Autodesk Inventor part; units mm, degrees
ref_plane "YZ Plane" through (0, 0, 0) normal (1, 0, 0) x (0, 1, 0)
ref_plane "XZ Plane" through (0, 0, 0) normal (0, 1, 0) x (-1, 0, 0)
ref_plane "XY Plane" through (0, 0, 0) normal (0, 0, 1) x (1, 0, 0)
sketch "Sketch1" plane through (0, 0, 0) normal (1, 0, 0) x (0, 1, 0)
  line L0 (-25, 24) -> (-25, -24)
  line L1 (-25, -24) -> (25, -24)
  line L2 (25, -24) -> (25, -22)
  line L3 (25, -22) -> (-23, -22)
  line L4 (-23, -22) -> (-23, 24)
  line L5 (-23, 24) -> (-25, 24)
extrude "Extrusion1" add sketch "Sketch1" along normal mid plane 131
sketch "Sketch2" plane through (65.5, 25, -24) normal (0, 0, -1) x (-1, 0, 0)
  circle A0 centre (41.4, -25) radius 3.5
  circle A1 centre (89.6, -25) radius 3.5
  line L0 (131, 0) -> (0, 0)
  line L1 (37.9, -25) -> (44.9, -25)
  line L2 (44.9, -25) -> (44.9, 0)
  line L3 (44.9, 0) -> (37.9, 0)
  line L4 (37.9, 0) -> (37.9, -25)
  line L5 (86.1, -25) -> (93.1, -25)
  line L6 (93.1, -25) -> (93.1, 0)
  line L7 (93.1, 0) -> (86.1, 0)
  line L8 (86.1, 0) -> (86.1, -25)
  line L9 (65.5, 0) -> (65.5, -8)
  circle A2 centre (65.5, -8) radius 4.75
  dimension "d17" = 7
  dimension "d18" = 7
  dimension "d129" = 8
  dimension "d130" = 9.5
hole "Hole1" at (24.1, 0, -24) at (-24.1, 0, -24) direction (0, 0, 1) diameter 7 depth 2
sketch "Sketch3" plane through (65.5, 25, -24) normal (0, 0, -1) x (-1, 0, 0)
  line L0 (65.5, -25) -> (14.2, -25)
  line L1 (65.5, -25) -> (116.8, -25)
  circle A0 centre (14.2, -25) radius 9.5
  circle A1 centre (14.2, -25) radius 1.75
  circle A2 centre (116.8, -25) radius 1.75
  dimension "d26" = 51.3
  dimension "d27" = 51.3
  dimension "d28" = 19
  dimension "d29" = 3.5
  dimension "d30" = 3.5
hole "Hole2" at (51.3, 0, -24) at (-51.3, 0, -24) direction (0, 0, 1) diameter 3.5 depth 2
sketch "Sketch7" plane through (65.5, 25, -24) normal (0, 0, -1) x (-1, 0, 0)
  circle A0 centre (14.2, -25) radius 1.75
  circle A1 centre (14.2, -25) radius 3.5
  point P0 (65.5, -25)
  dimension "d89" = 7
extrude "Extrusion3" cut sketch "Sketch7" against normal blind 2
sketch "Sketch8" plane through (65.5, 25, -24) normal (0, 0, -1) x (-1, 0, 0)
  circle A0 centre (14.2, -25) radius 3.5
  line L0 (14.2, -25) -> (39.2, -25) construction
  circle A1 centre (19.1497, -20.0503) radius 18.4
  circle A2 centre (19.1497, -20.0503) radius 15.5
  line L1 (14.2, -25) -> (19.1497, -20.0503)
  line L2 (19.1497, -20.0503) -> (36.8274, -2.3726)
  line L3 (36.8274, -2.3726) -> (1.4721, -37.7279)
  line L4 (6.139, -7.0395) -> (32.1605, -33.061)
  circle A3 centre (8.1896, -9.0901) radius 1.2
  circle A4 centre (30.1099, -31.0104) radius 1.2
  circle A5 centre (23.1614, -5.0784) radius 1.2
  circle A6 centre (4.1779, -24.0619) radius 1.2
  circle A7 centre (15.1381, -35.0221) radius 1.2
  circle A8 centre (34.1216, -16.0386) radius 1.2
  point P0 (65.5, -25)
  dimension "d96" = 31
  dimension "d97" = 25
  dimension "d98" = 180
  dimension "d99" = 50
  dimension "d100" = 2.4
  dimension "d101" = 2.4
  dimension "d104" = 2.4
  dimension "d105" = 2.4
  dimension "d106" = 2.4
  dimension "d107" = 2.4
extrude "Extrusion4" cut sketch "Sketch8" against normal blind 2 contours A3 A2 L4 | L4 A2 A3 | A4 A2 L4 | L4 A2 A4 | A6 A2 | A2 A6 | A7 A2 | A2 A7 | A8 A2 | A2 A8 | A5 A2 | A2 A5 | L4 A3 A2 | A2 A3 L4 | L4 A4 A2 | A2 A4 L4
sketch "Sketch9" plane through (65.5, 25, -24) normal (0, 0, -1) x (-1, 0, 0)
  circle A0 centre (34.1216, -16.0386) radius 1.2
  circle A1 centre (8.1896, -9.0901) radius 1.2
  circle A2 centre (15.1381, -35.0221) radius 1.2
  point P0 (65.5, -25)
extrude "Extrusion6" add sketch "Sketch9" against normal blind 2
sketch "Sketch11" plane through (65.5, 25, -24) normal (0, 0, -1) x (-1, 0, 0)
  circle A0 centre (4.1779, -24.0619) radius 1.2
  circle A1 centre (30.1099, -31.0104) radius 1.2
  circle A2 centre (23.1614, -5.0784) radius 1.2
  circle A3 centre (14.2, -25) radius 3.5
  circle A4 centre (116.8, -25) radius 1.75
  line L0 (65.5, -25) -> (65.5, 0)
  line L1 (0, 0) -> (131, 0)
  circle A5 centre (126.8221, -24.0619) radius 1.2
  circle A6 centre (100.8901, -31.0104) radius 1.2
  circle A7 centre (107.8386, -5.0784) radius 1.2
  circle A8 centre (116.8, -25) radius 3.5
extrude "Extrusion7" cut sketch "Sketch11" against normal blind 2 contours A5 | A6 | A7 | A8
sketch "Sketch12" plane through (65.5, 25, -24) normal (0, 0, -1) x (-1, 0, 0)
  circle A0 centre (116.8, -25) radius 3.5
  circle A1 centre (14.2, -25) radius 3.5
  circle A2 centre (14.2, -25) radius 6.5
  circle A3 centre (116.8, -25) radius 6.5
  point P0 (65.5, -25)
  dimension "d116" = 13
  dimension "d117" = 13
extrude "Extrusion8" cut sketch "Sketch12" against normal blind 2
extrude "Extrusion9" cut sketch "Sketch2" against normal blind 2 contours L1 A0 | L0 L6 A1 L8 | A0 L1 | A0 L4 L0 L2 | L5 A1 | A1 L5
fillet "Fillet1" radius 1 4 edges at (20.6, 25, -23) (27.6, 25, -23) (-20.6, 25, -23) (-27.6, 25, -23)
fillet "Fillet2" radius 1 2 edges at (65.5, 25, -23) (-65.5, 25, -23)
extrude "Extrusion10" cut sketch "Sketch2" against normal blind 2 contours A2
sketch "Sketch14" plane through (-65.5, -25, 24) normal (0, 0, 1) x (1, 0, 0)
  line L0 (0, 2) -> (131, 2)
  line L1 (131, 2) -> (131, 0)
  line L2 (131, 0) -> (0, 0)
  line L3 (0, 0) -> (0, 2)
  point P0 (65.5, 25)
extrude "Extrusion11" cut sketch "Sketch14" against normal blind 18
fillet "Fillet3" radius 1 2 edges at (-65.5, -24, 6) (65.5, -24, 6)
sketch "Sketch15" plane through (-65.5, -25, -24) normal (0, -1, 0) x (1, 0, 0)
  circle A0 centre (97.65, 20) radius 2
  circle A1 centre (33.35, 20) radius 2
  point P0 (65.5, 24)
  point P1 (131, 0)
  point P2 (0, 0)
  dimension "d139" = 4
  dimension "d140" = 4
extrude "Extrusion12" cut sketch "Sketch15" against normal blind 2
properties part number "drzak_motory"
Work out the finished part from the listing and answer in its coordinate system (mm). A direction names the side the tool comes from. Give positions to 0.01 mm unless a question says otherwise; leave off trailing zeros. Order: outer loops, then holes, each group sorted by start corner. A loop starts at its lowest first (then second) coordinate and runs counter-clockwise, first axis right, second up. Notation, with made-up numbers: (11, -7) -> (30, -7) arc R19 ccw to (30, 1) -> close; hole circle Ø2 at (33.5, 36.25). An arc over 180 degrees is marked (long way). Answer as CSV lines item,"result". Start each with the question number.
(1) Each of these flat-tipped pins is pushed along its axis until it touches: pin 1 Ø4 at (x, y) = (-1.5, 4.5) entering from +Z; pin 2 Ø1.5 at (x, z) = (21, -11.5) entering from +Y. Where does it stop, or does it pass through?
(2) Consider line 1 along Z through (x, y) = (32, -24); line 2 along Y through (x, z) = (-6, -10); line 3 along Z through (x, y) = (-49.5, -12.5). Determine where each line is inside the solid, lowest interval first.
(3) Which of the six approach directions +Z, -Z, +X, -X, +Y, -Y give full straight-line access (tool end or side, diameter ignored) to faces 1 (the cylindrical face through (-62.43, 0.48, -23.01)), 2 (the flat face through (-1, 1, -22))?
(4) Section C-C, the plane y = 11 is taken. Write down the section's boundary in (x, z), plus the area to 3 significant figures.
(5) Section B-B, the plane z = -4 is taken. Write down the section's boundary in (x, y), plus the area to 3 significant figures.
(6) Section A-A, the plane x = 0 is taken. Write down the section's boundary in (y, z), plus the area to 3 significant figures.
(7) For a pull along X with two mould halves and no side action, classify faces 3 (the flat face through (65.5, -7.9, -22.3)), 4 (the flat face through (-1, 0, -24)), 5 (the cylindrical face through (-34.19, -5.96, -23.01)) as released by +X, released by -X, zero draft, split by the parting line, or undercut.
(8) Section D-D, the plane y = 17 is taken. Write down the section's boundary in (x, z), plus the area to 3 significant figures.
Entries:
1,pin 1,"z = -22"
1,pin 2,"y = -23"
2,line 1,"-24 to -5.99, -2.01 to 6"
2,line 2,"-25 to -23"
2,line 3,"-24 to -22"
3,face 1,"+Z, -Z"
3,face 2,"+Z, +X, -X, +Y"
4,outline,"(-65.5, -24) -> (-27.6, -24) -> (-27.6, -22) -> (-65.5, -22) -> close; (-20.6, -24) -> (20.6, -24) -> (20.6, -22) -> (-20.6, -22) -> close; (27.6, -24) -> (65.5, -24) -> (65.5, -22) -> (27.6, -22) -> close"
4,area,"234 mm²"
5,outline,"(-65.5, -25) -> (-34.15, -25) -> (-34.15, -23) -> (-65.5, -23) -> close; (-30.15, -25) -> (30.15, -25) -> (30.15, -23) -> (-30.15, -23) -> close; (34.15, -25) -> (65.5, -25) -> (65.5, -23) -> (34.15, -23) -> close"
5,area,"246 mm²"
6,outline,"(-25, -24) -> (12.25, -24) -> (12.25, -22) -> (-23, -22) -> (-23, 6) -> (-25, 6) -> close; (21.75, -24) -> (25, -24) -> (25, -22) -> (21.75, -22) -> close"
6,area,"137 mm²"
7,face 3,"released by +X"
7,face 4,"zero draft"
7,face 5,"undercut"
8,outline,"(-65.5, -24) -> (-27.6, -24) -> (-27.6, -22) -> (-65.5, -22) -> close; (-20.6, -24) -> (-4.75, -24) -> (-4.75, -22) -> (-20.6, -22) -> close; (4.75, -24) -> (20.6, -24) -> (20.6, -22) -> (4.75, -22) -> close; (27.6, -24) -> (65.5, -24) -> (65.5, -22) -> (27.6, -22) -> close"
8,area,"215 mm²"
